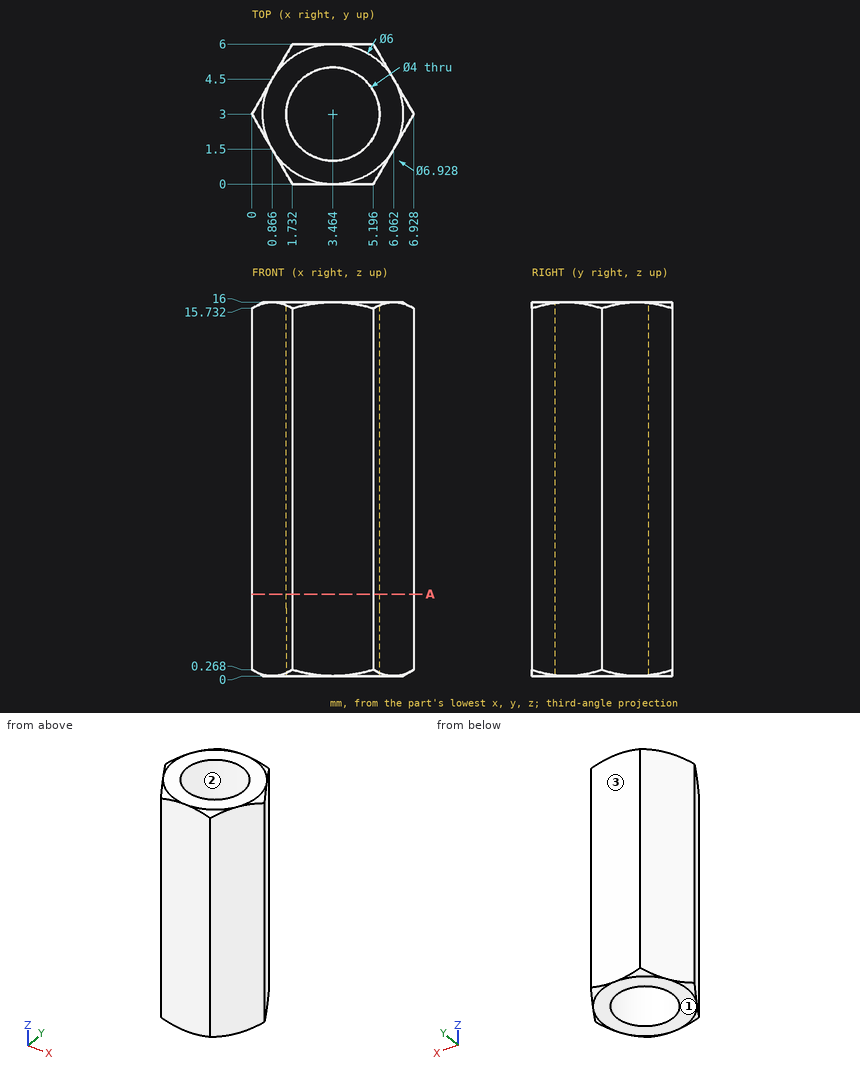
Part print with two shaded views. Sizes in mm from the minimum x, y, z corner. Coordinates: 2 decimals unless noted, no trailing zeros. Write each loop counter-clockwise with the first axis right and the second up, starting at its lowest first coordinate (ties: lowest second). Pieces come first, ordered by that corner, then holes. Notation, with made-up numbers: (-26, 6) - (19, 6) arc R20 ccw to (19, 40) - close; hole circle Ø1 at (-27, 52.5). An arc over 180 degrees is marked (long way). One line per item, written item: value. Start each with the question number.
1. Slice it at A-A (z = 3.5). Write the cut outline in (x, y), plus the area to 3 significant figures.
2. Mould opens along Y. For the marked faces 1, 2 and 3 say: released by +Y, released by -Y, zero draft, split by the parting line, or undercut.
3. Probe line 1 (Y direction, x = 2.25, z = 12.25); line 2 (X direction, y = 3.5, z = 3.75); line 3 (Y direction, x = 5, z = 4.25). List the from-to ranges inside material, lowest first. Write a range as from..to.
Answers below:
1. outline: (0, 3) - (1.73, 0) - (5.2, 0) - (6.93, 3) - (5.2, 6) - (1.73, 6) - close; hole circle Ø4 at (3.46, 3)
1. area: 18.6 mm^2
2. face 1: zero draft
2. face 2: undercut
2. face 3: released by +Y
3. line 1: y = 0..1.41, 4.59..6
3. line 2: x = 0.29..1.53, 5.4..6.64
3. line 3: y = 0..1.72, 4.28..6
